Read the model definition and answer for the solid it produces. Units are mm, in the model's axes. A direction names the side the tool comes from. Give positions to 0.01 mm unless a question says otherwise; leave off trailing zeros. Loops run counter-clockwise (first coordinate to the right, second up) from the corner with the lowest first, then second, coordinate; pieces in that order, holes last. Notation, with made-up numbers: (26, 23.25) - (84, 23.25) arc R22 ccw to (84, 50.25) - close; hole circle Ø4 at (-30, 33.5). An arc over 180 degrees is marked (long way). Use a Markdown table: item, result. Add a question column.
Item 1: A cutting plane is placed at D-D (z = -23). Determine the outline of the cut face in (x, y).
Item 2: Each of these flat-tipped pins is pushed along its axis until it touches: P1, Ø1.8, axis at y = 2.5, z = -24, coming from the -X side; P2, Ø0.9, axis at y = 67, z = -0.5, coming from the -X side; P3, Ø1, axis at x = -1, y = 22.5, coming from the -Z side. Where does it stop, or does it pass through?
Item 3: For a pull along Z with two mould halves and no side action, classify faces 6 (the face through (-3, 52, 0)), 7 (the face through (-18.6, 24.6, -18.6)), 8 (the face through (13.179, 24.65, 14.655)), 9 (the face through (-2.38, 50.99, 10.74)) as +Z half, -Z half, draft (parallel to the pull), parting line (faces both ways), or undercut.
Item 4: A cutting plane is placed at C-C (x = 0). Determine the outline of the cut face in (y, z), plus the area to 3 significant figures.
Item 5: A cutting plane is placed at A-A (x = -14.1). Determine the outline of the cut face in (y, z), plus the area to 3 significant figures.
Item 6: Consider probe 1 along Z at (x, y) = (-14.1, 14.5); probe 2 along X at (y, z) = (34, -15.5); probe 3 along X at (y, z) = (5, 16). Determine where each line is inside the solid, lowest interval first. Write a range as [from, to].
Item 7: Which of the six approach directions +Z, -Z, +X, -X, +Y, -Y give full straight-line access (tool end or side, diameter ignored) to faces 1 (the face through (10, 4, -24)), 2 (the face through (9, 50, 9)), 3 (the face through (-10, 4, -24)), 4 (the face through (-2, 64, 0)), 5 (the face through (13.179, 24.65, -16.345))?
Item 8: A cutting plane is placed at B-B (y = 24.5). Determine the outline of the cut face in (x, z).
from build123d import *

# Parameters (mm, degrees)
SKETCH_1_R      = 11
SKETCH_1_R_2    = 1.25
EXTRUDE_1_DEPTH = 50
SKETCH_1_3_R    = 11
SKETCH_1_3_R_2  = 2.5
EXTRUDE_2_DEPTH = 52
EXTRUDE_3_DEPTH = 72
EXTRUDE_4_DEPTH = 57
SKETCH_2_W      = 10
SKETCH_2_H      = 9
EXTRUDE_5_DEPTH = 6


with BuildPart() as part:
    # Sketch 1 → Extrude 1 (new body)
    with BuildSketch(Plane(origin=(0, 0, 0), x_dir=(1, 0, 0), z_dir=(0, 1, 0))):
        Polygon((-16.1, -21.1), (16.1, -21.1), (21.1, -16.1), (21.1, 16.1), (16.1, 21.1), (-16.1, 21.1), (-21.1, 16.1), (-21.1, -16.1), align=None)
        Circle(SKETCH_1_R, mode=Mode.SUBTRACT)
        with Locations((-14.1, 15.5)):
            Circle(SKETCH_1_R_2, mode=Mode.SUBTRACT)
        with Locations((14.1, 15.5)):
            Circle(SKETCH_1_R_2, mode=Mode.SUBTRACT)
        with Locations((14.1, -15.5)):
            Circle(SKETCH_1_R_2, mode=Mode.SUBTRACT)
        with Locations((-14.1, -15.5)):
            Circle(SKETCH_1_R_2, mode=Mode.SUBTRACT)
    extrude(amount=EXTRUDE_1_DEPTH)

    # Sketch 1_3 → Extrude 2 (add)
    with BuildSketch(Plane(origin=(0, 0, 0), x_dir=(1, 0, 0), z_dir=(0, 1, 0))):
        Circle(SKETCH_1_3_R)
        Circle(SKETCH_1_3_R_2, mode=Mode.SUBTRACT)
    extrude(amount=EXTRUDE_2_DEPTH)

    # Sketch 1_4 → Extrude 3 (add)
    with BuildSketch(Plane(origin=(0, 0, 0), x_dir=(1, 0, 0), z_dir=(0, 1, 0))):
        with BuildLine():
            ThreePointArc((2.5, 0), (0.790569415, 2.371708245), (-2, 1.5))
            Line((-2, 1.5), (-2, -1.5))
            ThreePointArc((-2, -1.5), (0.790569415, -2.371708245), (2.5, 0))
        make_face()
    extrude(amount=EXTRUDE_3_DEPTH)

    # Sketch 1_5 → Extrude 4 (add)
    with BuildSketch(Plane(origin=(0, 0, 0), x_dir=(1, 0, 0), z_dir=(0, 1, 0))):
        with BuildLine():
            ThreePointArc((2.5, 0), (0.790569415, 2.371708245), (-2, 1.5))
            Line((-2, 1.5), (-2, -1.5))
            ThreePointArc((-2, -1.5), (0.790569415, -2.371708245), (2.5, 0))
        make_face()
        with BuildLine():
            Line((-2, -1.5), (-2, 1.5))
            ThreePointArc((-2, 1.5), (-2.5, 0), (-2, -1.5))
        make_face()
    extrude(amount=EXTRUDE_4_DEPTH)

    # Sketch 2 → Extrude 5 (add)
    with BuildSketch(Plane(origin=(0, 0, -21.1), x_dir=(-1, 0, 0), z_dir=(0, 0, -1))):
        with Locations((5, 4.5)):
            Rectangle(SKETCH_2_W, SKETCH_2_H)
        with Locations((-5, 4.5)):
            Rectangle(SKETCH_2_W, SKETCH_2_H)
    extrude(amount=EXTRUDE_5_DEPTH)


solid = part.part
Geometry says:
| question | item | result |
|---|---|---|
| 1 | outline | (-10, 0) - (10, 0) - (10, 9) - (-10, 9) - close |
| 2 | P1 | x = -10 |
| 2 | P2 | x = -2 |
| 2 | P3 | z = -21.1 |
| 3 | face 6 | draft |
| 3 | face 7 | -Z half |
| 3 | face 8 | undercut |
| 3 | face 9 | parting line |
| 4 | outline | (0, -27.1) - (9, -27.1) - (9, -21.1) - (50, -21.1) - (50, -11) - (52, -11) - (52, -2.5) - (72, -2.5) - (72, 2.5) - (52, 2.5) - (52, 11) - (50, 11) - (50, 21.1) - (0, 21.1) - close |
| 4 | area | 2,310 mm² |
| 5 | outline | (0, -21.1) - (50, -21.1) - (50, -16.75) - (0, -16.75) - close; (0, -14.25) - (50, -14.25) - (50, 14.25) - (0, 14.25) - close; (0, 16.75) - (50, 16.75) - (50, 21.1) - (0, 21.1) - close |
| 5 | area | 1,860 mm² |
| 6 | probe 1 | [-21.1, -16.75], [-14.25, 14.25], [16.75, 21.1] |
| 6 | probe 2 | [-21.1, -15.35], [-12.85, 12.85], [15.35, 21.1] |
| 6 | probe 3 | [-21.1, -15.25], [-12.95, 12.95], [15.25, 21.1] |
| 7 | face 1 | -Z, +X, +Y, -Y |
| 7 | face 2 | +Y |
| 7 | face 3 | -Z, -X, +Y, -Y |
| 7 | face 4 | +Z, -Z, -X, +Y |
| 7 | face 5 | +Y, -Y |
| 8 | outline | (-21.1, -16.1) - (-16.1, -21.1) - (16.1, -21.1) - (21.1, -16.1) - (21.1, 16.1) - (16.1, 21.1) - (-16.1, 21.1) - (-21.1, 16.1) - close; hole circle Ø2.5 at (-14.1, -15.5); hole circle Ø2.5 at (-14.1, 15.5); hole circle Ø2.5 at (14.1, -15.5); hole circle Ø2.5 at (14.1, 15.5) |
